Model file for the job. Use its own axes, mm. Face numbers are marked on the shaded views. A direction names the side the tool comes from. Coordinates: 2 decimals unless noted, no trailing zeros. Loops run counter-clockwise (first coordinate to the right, second up) from the corner with the lowest first, then second, coordinate; pieces in that order, holes last.
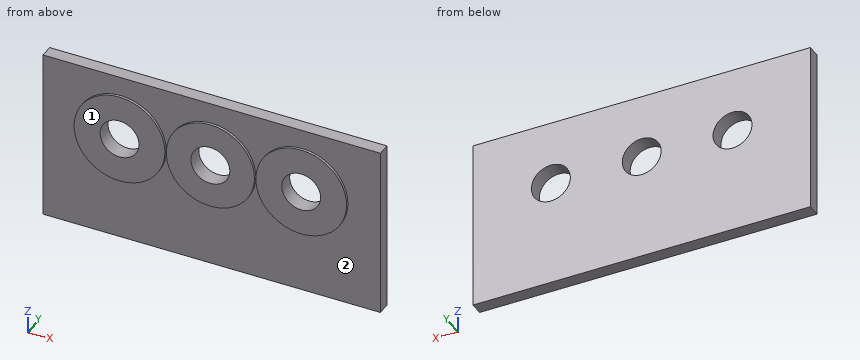
from build123d import *

# Parameters (mm, degrees)
F0_W     = 130
F0_H     = 66.465674
F0_R     = 17.5
F0_R_2   = 7.5
F0_R_3   = 17
F1_DEPTH = 5
F2_DEPTH = 6
F3_DEPTH = 6
F4_DEPTH = 6


with BuildPart() as f1:
    # F0 (on Front) → F1 (new body)
    with BuildSketch(Plane.XZ):
        Rectangle(F0_W, F0_H)
        with Locations((-35, 8.232837)):
            Circle(F0_R, mode=Mode.SUBTRACT)
        with BuildLine():
            ThreePointArc((-17.5, 8.232837), (0, 25.732837), (17.5, 8.232837))
            ThreePointArc((17.5, 8.232837), (0, -9.267163), (-17.5, 8.232837))
        make_face(mode=Mode.SUBTRACT)
        with BuildLine():
            ThreePointArc((17.5, 8.232837), (35, 25.732837), (52.5, 8.232837))
            ThreePointArc((52.5, 8.232837), (35, -9.267163), (17.5, 8.232837))
        make_face(mode=Mode.SUBTRACT)
        with Locations((-35, 8.232837)):
            Circle(F0_R)
        with Locations((-35, 8.232837)):
            Circle(F0_R_2, mode=Mode.SUBTRACT)
        with BuildLine():
            ThreePointArc((-17.5, 8.232837), (0, -9.267163), (17.5, 8.232837))
            ThreePointArc((17.5, 8.232837), (0, 25.732837), (-17.5, 8.232837))
        make_face()
        with Locations((0, 8.232837)):
            Circle(F0_R_3, mode=Mode.SUBTRACT)
        with BuildLine():
            ThreePointArc((17.5, 8.232837), (35, -9.267163), (52.5, 8.232837))
            ThreePointArc((52.5, 8.232837), (35, 25.732837), (17.5, 8.232837))
        make_face()
        with Locations((35, 8.232837)):
            Circle(F0_R_2, mode=Mode.SUBTRACT)
        with Locations((0, 8.232837)):
            Circle(F0_R_3)
        with Locations((0, 8.232837)):
            Circle(F0_R_2, mode=Mode.SUBTRACT)
    extrude(amount=F1_DEPTH)

    # F0 (on Front) → F2 (join)
    with BuildSketch(Plane.XZ):
        with BuildLine():
            ThreePointArc((17.5, 8.232837), (35, -9.267163), (52.5, 8.232837))
            ThreePointArc((52.5, 8.232837), (35, 25.732837), (17.5, 8.232837))
        make_face()
        with Locations((35, 8.232837)):
            Circle(F0_R_2, mode=Mode.SUBTRACT)
    extrude(amount=F2_DEPTH)

    # F0 (on Front) → F3 (join)
    with BuildSketch(Plane.XZ):
        with Locations((-35, 8.232837)):
            Circle(F0_R)
        with Locations((-35, 8.232837)):
            Circle(F0_R_2, mode=Mode.SUBTRACT)
    extrude(amount=F3_DEPTH)

    # F0 (on Front) → F4 (join)
    with BuildSketch(Plane.XZ):
        with Locations((0, 8.232837)):
            Circle(F0_R_3)
        with Locations((0, 8.232837)):
            Circle(F0_R_2, mode=Mode.SUBTRACT)
    extrude(amount=F4_DEPTH)


solid = f1.part
Q1. Slice it at A-A (x = 0). List the corners of the cut face in (y, z), and give its area (3 significant figures).
Answers:
outline: (-6, -8.77) - (-5, -8.77) - (-5, -33.23) - (0, -33.23) - (0, 0.73) - (-6, 0.73) - close; (-6, 15.73) - (0, 15.73) - (0, 33.23) - (-5, 33.23) - (-5, 25.23) - (-6, 25.23) - close
area: 276 mm2
Q2. Slice it at C-C (x = -30). List the corners of the cut face in (y, z), and give its area (3 significant figures).
Answers:
outline: (-6, -8.54) - (-5, -8.54) - (-5, -33.23) - (0, -33.23) - (0, 2.64) - (-6, 2.64) - close; (-6, 13.82) - (0, 13.82) - (0, 33.23) - (-5, 33.23) - (-5, 25) - (-6, 25) - close
area: 299 mm2
Q3. Drill centre lines: line 1 (Z direction, x = 35, y = -4.1); line 2 (X direction, y = -3.4, z = 6.5); line 3 (Y direction, x = -47, z = 21). Where is each one in solid material? Low to high.
Answers:
line 1: z = -33.23 to 0.73, 15.73 to 33.23
line 2: x = -65 to -42.3, -27.7 to -7.3, 7.3 to 27.7, 42.3 to 65
line 3: y = -5 to 0
Q4. Slice it at D-D (z = -11.5). List the corners of the cut face in (x, y), and give its area (3 significant figures).
Answers:
outline: (-65, -5) - (65, -5) - (65, 0) - (-65, 0) - close
area: 650 mm2
Q5. Slice it at B-B (z = 4). List the corners of the cut face in (x, y), and give its area (3 significant figures).
Answers:
outline: (-65, -5) - (-51.98, -5) - (-51.98, -6) - (-41.19, -6) - (-41.19, 0) - (-65, 0) - close; (-28.81, -6) - (-18.02, -6) - (-18.02, -5) - (-16.46, -5) - (-16.46, -6) - (-6.19, -6) - (-6.19, 0) - (-28.81, 0) - close; (6.19, -6) - (16.46, -6) - (16.46, -5) - (18.02, -5) - (18.02, -6) - (28.81, -6) - (28.81, 0) - (6.19, 0) - close; (41.19, -6) - (51.98, -6) - (51.98, -5) - (65, -5) - (65, 0) - (41.19, 0) - close
area: 528 mm2
Q6. Which spindle directions (+Z, -Z, +X, -X, +Y, -Y) get a long thin tool onto all of the face, cutting with end or side? Do the marked faces 1 and 2. Say none if no direction does.
Answers:
face 1: +Z, -Z, +X, -X, -Y
face 2: -Y
